The listing builds one solid part. Answer for the finished solid, in the listing's coordinates (mm). A direction names the side the tool comes from. Coordinates: 2 decimals unless noted, no trailing zeros. Write each loop counter-clockwise with the first axis right and the second up, starting at its lowest first coordinate (ties: lowest second). Pieces come first, ordered by that corner, then holes.
from build123d import *

# Parameters (mm, degrees)
F0_R     = 4
F0_R_2   = 8
F1_DEPTH = 6
F2_R     = 5
F3_R     = 5
F4_R     = 3


with BuildPart() as f1:
    # F0 (on Front) → F1 (new body)
    with BuildSketch(Plane.XZ):
        with BuildLine():
            Line((-67.0491158962, 8.89), (-67.0491158962, 0))
            Line((-67.0491158962, 0), (72.6508841038, 0))
            Line((72.6508841038, 0), (72.6508841038, 25.4))
            Line((72.6508841038, 25.4), (63.9108841038, 25.4))
            ThreePointArc((63.9108841038, 25.4), (57.4108841038, 18.9), (50.9108841038, 25.4))
            ThreePointArc((50.9108841038, 25.4), (51.9554394899, 28.933853996), (54.7533838162, 31.3319214612))
            Line((54.7533838162, 31.3319214612), (72.6508841038, 39.35))
            Line((72.6508841038, 39.35), (72.6508841038, 50.8))
            Line((72.6508841038, 50.8), (47.2508841038, 50.8))
            Line((47.2508841038, 50.8), (21.8508841038, 50.8))
            Line((21.8508841038, 50.8), (-22.5991158962, 50.8))
            Line((-22.5991158962, 50.8), (-67.0491158962, 50.8))
            Line((-67.0491158962, 50.8), (-67.0491158962, 41.91))
            Line((-67.0491158962, 41.91), (-67.0491158962, 8.89))
        make_face()
        with Locations((-58.1591158962, 8.89)):
            Circle(F0_R, mode=Mode.SUBTRACT)
        with Locations((-47.9991158962, 25.4)):
            Circle(F0_R_2, mode=Mode.SUBTRACT)
        with Locations((63.7608841038, 8.89)):
            Circle(F0_R, mode=Mode.SUBTRACT)
        with Locations((-22.5991158962, 33.02)):
            Circle(F0_R, mode=Mode.SUBTRACT)
        with Locations((-58.1591158962, 41.91)):
            Circle(F0_R, mode=Mode.SUBTRACT)
        with Locations((21.8508841038, 43.18)):
            Circle(F0_R, mode=Mode.SUBTRACT)
        with Locations((47.2508841038, 40.64)):
            Circle(F0_R, mode=Mode.SUBTRACT)
    extrude(amount=F1_DEPTH)

    # F2
    f2_edges = [f1.edges().sort_by_distance(p)[0] for p in [
        (-67.049116, -3, 50.8),
        (-67.049116, -3, 0),
        (72.650884, -3, 0),
    ]]
    fillet(f2_edges, radius=F2_R)

    # F3
    f3_edges = [f1.edges().sort_by_distance(p)[0] for p in [
        (72.650884, -3, 50.8),
    ]]
    fillet(f3_edges, radius=F3_R)

    # F4
    f4_edges = [f1.edges().sort_by_distance(p)[0] for p in [
        (63.910884, -3, 25.4),
    ]]
    fillet(f4_edges, radius=F4_R)


solid = f1.part
Q1. The part is cut by section A-A, the plane z = 8.89. Write down the section's boundary in (x, y).
Answers below:
outline: (-67.05, -6) - (-62.16, -6) - (-62.16, 0) - (-67.05, 0) - close; (-54.16, -6) - (59.76, -6) - (59.76, 0) - (-54.16, 0) - close; (67.76, -6) - (72.65, -6) - (72.65, 0) - (67.76, 0) - close
Q2. Which of the six approach directions +Z, -Z, +X, -X, +Y, -Y give full straight-line access (tool end or side, diameter ignored) to faces 4 (the face through (64.65, -3.04, 24.82)), 5 (the face through (-67.049, -3, 26)), 6 (the face through (70, -3, 25.4))?
Answers below:
face 4: +Y, -Y
face 5: +Z, -Z, -X, +Y, -Y
face 6: +X, +Y, -Y
Q3. The part is cut by section B-B, the plane x = 49.5. Write down the section's boundary in (y, z).
Answers below:
outline: (-6, 0) - (0, 0) - (0, 37.33) - (-6, 37.33) - close; (-6, 43.95) - (0, 43.95) - (0, 50.8) - (-6, 50.8) - close
Q4. The part is cut by section C-C, the plane y = -2.8. Write down the section's boundary in (x, z).
Answers below:
outline: (-67.05, 5) arc R5 ccw to (-62.05, 0) - (67.65, 0) arc R5 ccw to (72.65, 5) - (72.65, 25.4) - (66.42, 25.4) arc R3 ccw to (63.58, 23.35) arc R6.5 cw (long way) to (54.75, 31.33) - (72.65, 39.35) - (72.65, 45.8) arc R5 ccw to (67.65, 50.8) - (-62.05, 50.8) arc R5 ccw to (-67.05, 45.8) - close; hole circle Ø8 at (-58.16, 8.89); hole circle Ø8 at (-58.16, 41.91); hole circle Ø16 at (-48, 25.4); hole circle Ø8 at (-22.6, 33.02); hole circle Ø8 at (21.85, 43.18); hole circle Ø8 at (47.25, 40.64); hole circle Ø8 at (63.76, 8.89)
Q5. The part is cut by section D-D, the plane z = 40.64. Write down the section's boundary in (x, y), then the cut area to 3 significant figures.
Answers below:
outline: (-67.05, -6) - (-61.95, -6) - (-61.95, 0) - (-67.05, 0) - close; (-54.37, -6) - (18.76, -6) - (18.76, 0) - (-54.37, 0) - close; (24.94, -6) - (43.25, -6) - (43.25, 0) - (24.94, 0) - close; (51.25, -6) - (72.65, -6) - (72.65, 0) - (51.25, 0) - close
area: 708 mm2
Q6. Given pin 1 (3 mm diameter, centred on x = 70.5, y = -1.5, fed in from +Z), flat-ended and moving along its own axis, determine where the tip first touches the part or whether it passes through.
Answers below:
pin 1: stops at z = 50.61
Q7. Determine the mould class of faces 1 (the face through (71.15, -3.04, 1.43)), 2 (the face through (63.577, -2.958, 35.285)), 3 (the face through (72.651, -3, 15)) for opening direction Z: released by +Z, released by -Z, zero draft, split by the parting line, or undercut.
Answers below:
face 1: released by -Z
face 2: undercut
face 3: zero draft
Q8. Find the intervals of material crossed by probe 1 along X at (y, z) = (-2.35, 9.5); probe 2 along X at (y, z) = (-2.85, 12.5); probe 3 along Z at (x, y) = (66.5, -2.25) (3 decimals), in increasing order.
Answers below:
probe 1: x = -67.05 to -62.11, -54.21 to 59.81, 67.71 to 72.65
probe 2: x = -67.05 to -59.88, -56.44 to 62.04, 65.48 to 72.65
probe 3: z = 0 to 5.975, 11.805 to 25.4, 36.594 to 50.8
